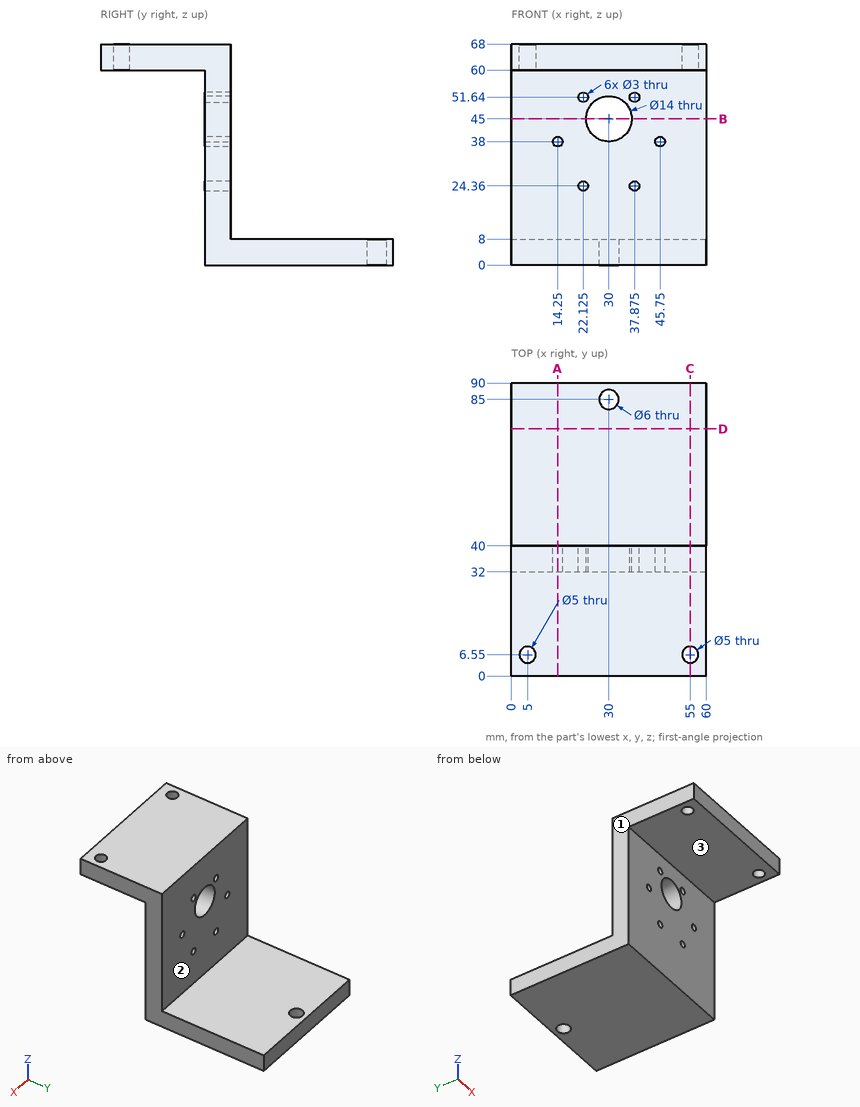
Part print with two shaded views. Sizes in mm from the minimum x, y, z corner. A direction names the side the tool comes from. Round coordinates to 2 decimals unless told otherwise and drop trailing zeros. Write each loop counter-clockwise with the first axis right and the second up, starting at its lowest first coordinate (ties: lowest second). Pieces come first, ordered by that corner, then holes. Notation, with made-up numbers: M 15.25,11 L 20.25,11 A12 ccw 20.25,17 Z; hole C -32,3 d2. An arc over 180 degrees is marked long. Put each result on its own line as item: value. Start each with the question number.
1) Saw through at D-D, the plane y = 76. Write the cut outline in (x, z).
2) Drill centre lines: probe 1 along Z at (x, y) = (38, 39.5) (1 decimal); probe 2 along X at (y, z) = (5, 62); probe 3 along Z at (x, y) = (54, 23). Where is each one in solid material? Low to high. Write a range as [from, to].
3) Saw through at C-C, the plane x = 55. Write the cut outline in (y, z).
4) Saw through at A-A, the plane x = 14.25. Write the cut outline in (y, z).
5) Pin check, flat tips, straight feed: pin 1 Ø6 at (x, z) = (33.5, 54) entering from +Y; pin 2 Ø16 at (x, y) = (18, 22) entering from -Z; pin 3 Ø4.5 at (x, y) = (5, 6.55) entering from +Z; pin 4 Ø2 at (x, z) = (27, 30) entering from -Y. Stop position of each tip, or through.
6) Saw through at B-B, the plane z = 45. Write the cut outline in (x, y), and give its area (3 significant figures).
7) 3-axis set-ups, long thin cutter, end or side, ignore diameter. For the marked faces 1, 2 and 3: which of +Z, -Z, +X, -X, +Y, -Y reach the whole face in a straight line?
Resolved:
1. outline: M 0,0 L 60,0 L 60,8 L 0,8 Z
2. probe 1: [0, 22.9], [25.9, 50.1], [53.1, 68]
2. probe 2: [0, 3.04], [6.96, 53.04], [56.96, 60]
2. probe 3: [60, 68]
3. outline: M 0,60 L 4.05,60 L 4.05,68 L 0,68 Z; M 9.05,60 L 32,60 L 32,0 L 90,0 L 90,8 L 40,8 L 40,68 L 9.05,68 Z
4. outline: M 0,60 L 32,60 L 32,39.5 L 40,39.5 L 40,68 L 0,68 Z; M 32,0 L 90,0 L 90,8 L 40,8 L 40,36.5 L 32,36.5 Z
5. pin 1: y = 40
5. pin 2: z = 60
5. pin 3: through
5. pin 4: y = 32
6. outline: M 0,32 L 23,32 L 23,40 L 0,40 Z; M 37,32 L 60,32 L 60,40 L 37,40 Z
6. area: 368 mm²
7. face 1: +Z, -Z, -X, +Y, -Y
7. face 2: +Z, +X, -X, +Y
7. face 3: -Z, +X, -X, -Y
